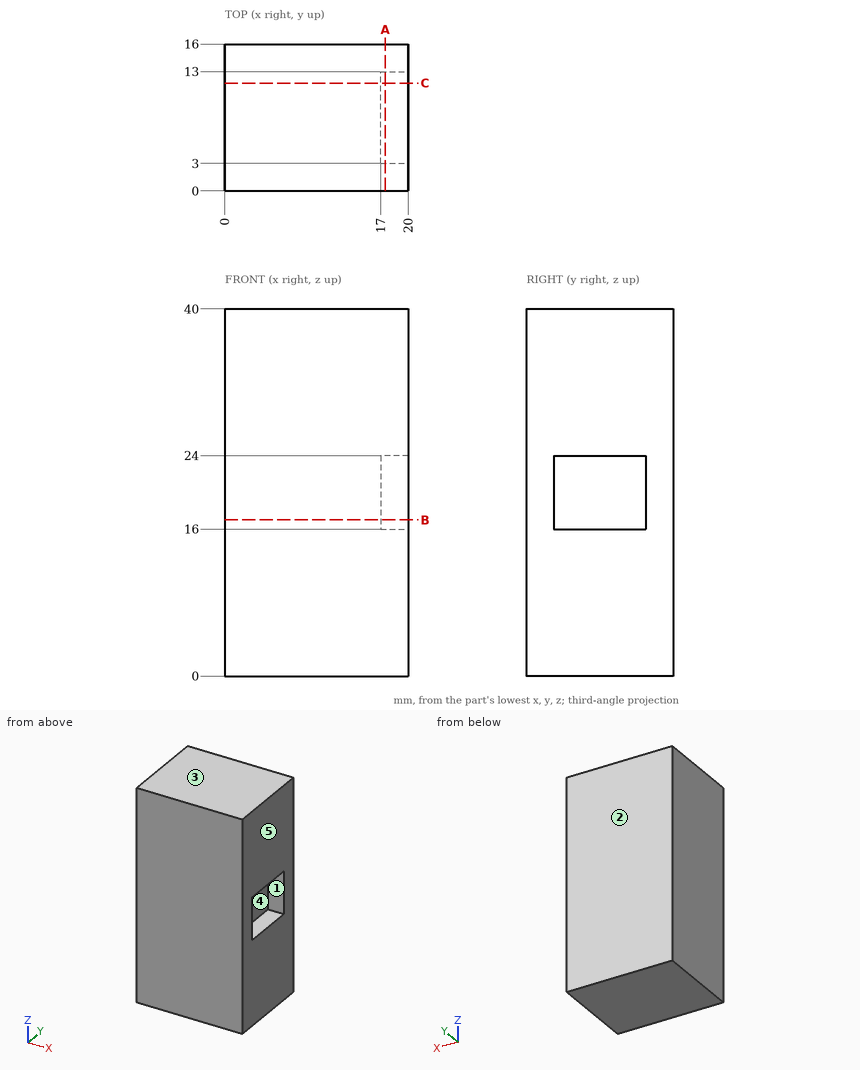
The drawing under review shows one solid part. Ordinate dimensions are in mm from its lowest x, y, z. A direction names the side the tool comes from. Coordinates: 2 decimals unless noted, no trailing zeros. Write each loop counter-clockwise with the first axis right and the second up, starting at its lowest first coordinate (ties: lowest second). Pieces come first, ordered by that corner, then holes.
1) Add section A-A (x = 17.5). Write out the cut boundary in (y, z).
2) Add section C-C (y = 11.75). Write out the cut boundary in (x, z), plus the area to 3 significant figures.
3) Machinability: for the marked faces 1 and 2, which of the approach directions +Z, -Z, +X, -X, +Y, -Y give a long, thin tool a straight path to every point of the face, cutting with its end or side? Answer none if there is none.
4) Mouldability with a two-part tool opening along Z and no side actions: class the marked faces 3, 4 and 5 as +Z half, -Z half, draft (parallel to the pull), parting line (faces both ways), or undercut.
5) Add section B-B (z = 17). Write out the cut boundary in (x, y), plus the area to 3 significant figures.
6) To check wall thickness, follow L1, parallel to Z at x = 18.5, y = 4.75; L2, parallel to X at y = 9.5, z = 21.5. State the ranges of each line that lie inside material, in increasing order.
7) Insertion check: pin 1 (3 mm diameter, centred on y = 5.5, z = 19.5, fed in from +X). The pin has a flat end and moves straight along its axis. Give the tip position at first contact, or say it passes through.
Check result:
1. outline: (0, 0) - (16, 0) - (16, 40) - (0, 40) - close; hole (3, 16) - (13, 16) - (13, 24) - (3, 24) - close
2. outline: (0, 0) - (20, 0) - (20, 16) - (17, 16) - (17, 24) - (20, 24) - (20, 40) - (0, 40) - close
2. area: 776 mm2
3. face 1: +X
3. face 2: +Z, -Z, +X, -X, +Y
4. face 3: +Z half
4. face 4: undercut
4. face 5: draft
5. outline: (0, 0) - (20, 0) - (20, 3) - (17, 3) - (17, 13) - (20, 13) - (20, 16) - (0, 16) - close
5. area: 290 mm2
6. L1: z = 0 to 16, 24 to 40
6. L2: x = 0 to 17
7. pin 1: stops at x = 17
